```python
from build123d import *

# Parameters (mm, degrees)
PAD023_DEPTH = 18
SKETCH049_R  = 1.4
PAD024_DEPTH = 14
PAD025_DEPTH = 18


with BuildPart() as part:
    # Sketch046 → Pad023 (new body)
    with BuildSketch(Plane.XY.offset(8.5)):
        with BuildLine():
            ThreePointArc((1.041889, -5.908847), (6, 0), (1.041889, 5.908847))
            Line((1.128713, 6.40125), (1.041889, 5.908847))
            ThreePointArc((1.128713, -6.40125), (6.5, 0), (1.128713, 6.40125))
            Line((1.128713, -6.40125), (1.041889, -5.908847))
        make_face()
    extrude(amount=PAD023_DEPTH)

    # Sketch049 (on DatumPlane) → Pad024 (join)
    with BuildSketch(Plane(origin=(6, 0, 26.5), x_dir=(0, 1, 0), z_dir=(1, 0, 0))):
        with Locations((0, -9)):
            Circle(SKETCH049_R)
    extrude(amount=PAD024_DEPTH)

    # Sketch050 → Pad025 (join)
    with BuildSketch(Plane.XY.offset(8.5)):
        with BuildLine():
            ThreePointArc((1.745858, -9.90125), (10.053993, 0), (1.745858, 9.90125))
            Line((1.832682, 10.393654), (1.745858, 9.90125))
            ThreePointArc((1.832682, -10.393654), (10.553993, 0), (1.832682, 10.393654))
            Line((1.832682, -10.393654), (1.745858, -9.90125))
        make_face()
    extrude(amount=PAD025_DEPTH)


solid = part.part
```
Source: CAD feature listing. Evaluate the final solid. Frame: model axes, mm. A direction names the side the tool comes from. Give positions to 0.01 mm unless a question says otherwise; leave off trailing zeros. Loops run counter-clockwise (first coordinate to the right, second up) from the corner with the lowest first, then second, coordinate; pieces in that order, holes last. Notation, with made-up numbers: M 76.5,73.5 L 93.5,73.5 A36 ccw 93.5,110.5 Z; hole C 86,38 d6. An arc over 180 degrees is marked long. Put each result on its own line as item: value.
Q1. Section D-D (x = 14). Return the cut outline in (y, z), and give its area (3 significant figures).
Response values:
outline: C 0,17.5 d2.8
area: 6.16 mm²
Q2. Reachability of faces 4 (the cylindrical face through (8.174, -0.303, 16.133)), 5 (the cylindrical face through (15.162, -0.303, 16.133)), 6 (the flat face through (10.4, 0, 8.5)) from +Z, -Z, +X, -X, +Y, -Y: full face, straight path, thin tool, end or side. Return the list, or none.
Response values:
face 4: none
face 5: +X
face 6: -Z, +X, -X, +Y, -Y
Q3. Line query: probe 1 along Y at (x, z) = (2.25, 24); probe 2 along Y at (x, z) = (2, 10.25); probe 3 along X at (y, z) = (3.5, 19.5). Output: solid intervals per line, ascending. Write a range as [from, to].
Response values:
probe 1: y = [-10.31, -9.8], [-6.1, -5.56], [5.56, 6.1], [9.8, 10.31]
probe 2: y = [-10.36, -9.85], [-6.18, -5.66], [5.66, 6.18], [9.85, 10.36]
probe 3: x = [4.87, 5.48], [9.43, 9.96]
Q4. Mould query, pull axis Y, two halves, no side actions, for faces 1 (the flat face through (6.2, 0, 26.5)), 2 (the cylindrical face through (10.55, -0.21, 19.37)), 3 (the cylindrical face through (10.052, -0.197, 19.374)). Classes: released by +Y, released by -Y, zero draft, split by the parting line, or undercut.
Response values:
face 1: zero draft
face 2: split by the parting line
face 3: undercut
Q5. Section A-A (z = 22.25). Return the cut outline in (x, y), and give its area (3 significant figures).
Response values:
outline: M 1.04,-5.91 L 1.13,-6.4 A6.5 ccw 1.13,6.4 L 1.04,5.91 A6 cw Z; M 1.75,-9.9 L 1.83,-10.39 A10.55 ccw 1.83,10.39 L 1.75,9.9 A10.05 cw Z
area: 23.1 mm²
Q6. Pin query (flat end, axial travel): P1, Ø5, axis at x = 5.5, z = 23, coming from the -Y side; P2, Ø4, axis at x = 9.5, y = 6.5, coming from the +Z side; P3, Ø1.5, axis at x = 8.5, z = 13, coming from the -Y side; P4, Ø1.5, axis at y = 4.5, z = 13.5, coming from the +X side. Return the tip coordinate at first contact, or that it passes through.
Response values:
P1: stops at y = -10.12
P2: stops at z = 26.5
P3: stops at y = -7.16
P4: stops at x = 9.87
Q7. Section B-B (y = 0). Return the cut outline in (x, z), and give its area (3 significant figures).
Response values:
outline: M 6,8.5 L 6.5,8.5 L 6.5,16.1 L 10.05,16.1 L 10.05,8.5 L 10.55,8.5 L 10.55,16.1 L 20,16.1 L 20,18.9 L 10.55,18.9 L 10.55,26.5 L 10.05,26.5 L 10.05,18.9 L 6.5,18.9 L 6.5,26.5 L 6,26.5 Z
area: 54.4 mm²
Q8. Section C-C (y = -5). Return the cut outline in (x, z).
Response values:
outline: M 3.32,8.5 L 4.15,8.5 L 4.15,26.5 L 3.32,26.5 Z; M 8.72,8.5 L 9.29,8.5 L 9.29,26.5 L 8.72,26.5 Z
